Here's how the part is built. I have some questions about the finished solid (model axes, mm). Face numbers are marked on the shaded views. A direction names the side the tool comes from. Coordinates: 2 decimals unless noted, no trailing zeros. Order: outer loops, then holes, each group sorted by start corner. A loop starts at its lowest first (then second) coordinate and runs counter-clockwise, first axis right, second up. Notation, with made-up numbers: (58.5, 20.5) - (93.5, 20.5) arc R23 cw to (93.5, 28.5) - close; hole circle Ø4 at (-14.75, 59.25). An arc over 180 degrees is marked (long way). Answer in a Markdown table with one row per item. Add a question column.
Item 1: I want a section at C-C (x = 9). Please give me the cut outline in (y, z), plus the area to 3 significant figures.
Item 2: Will these pins go through, and if not, where does the flat tip stop? pin 1 Ø4 at (x, y) = (2.5, 3) entering from -Z; pin 2 Ø1.5 at (x, y) = (11, 12.5) entering from +Z; pin 3 Ø2 at (y, z) = (7, 5) entering from -X; pin 4 Ø5 at (x, z) = (13.5, 24) entering from -Y.
Item 3: I want a section at A-A (y = 0). Please give me the cut outline in (x, z) (3 decimals).
Item 4: Thinking about a two-plate mould opening in Z: for the marked faces 4, 5 and 6, which applies, +Z half, -Z half, draft (parallel to the pull), parting line (faces both ways), or undercut?
Item 5: If I drill on line 1 along Z through (x, y) = (-7, -14); line 2 along Y through (x, z) = (0, 24) (3 decimals); line 3 along Z through (x, y) = (7.5, -9), over which ranges is the centre line in solid material (lowest first)? Write a range as from..to.
Item 6: On a 3-axis mill with a long thin cutter (end or side, diameter ignored), from which of +Z, -Z, +X, -X, +Y, -Y can I reach the whole of each face in a straight line? I mean the marked faces 1, 2 and 3. Say none if no direction works.
Item 7: I want a section at D-D (z = 11.5). Please give me the cut outline in (x, y) (3 decimals), plus the area to 3 significant figures.
```python
from build123d import *

# Parameters (mm, degrees)
SZKIC1_R                    = 15.345
DODANIE_WYCI_GNI_CIE1_DEPTH = 30.5
SZKIC2_R                    = 11.5
DODANIE_WYCI_GNI_CIE2_DEPTH = 5.5
SZKIC3_R                    = 18
DODANIE_WYCI_GNI_CIE3_DEPTH = 0.5
SZKIC9_R                    = 18
DODANIE_WYCI_GNI_CIE6_DEPTH = 0.5
SZKIC6_R                    = 7
WYTNIJ_WYCI_GNI_CIE1_DEPTH  = 37


with BuildPart() as part:
    # Szkic1 → Dodanie-wyciągnięcie1 (new body)
    with BuildSketch(Plane.XY):
        Circle(SZKIC1_R)
    extrude(amount=DODANIE_WYCI_GNI_CIE1_DEPTH)

    # Szkic2 → Dodanie-wyciągnięcie2 (add)
    with BuildSketch(Plane.XY.offset(30.5)):
        Circle(SZKIC2_R)
    extrude(amount=DODANIE_WYCI_GNI_CIE2_DEPTH)

    # Szkic3 → Dodanie-wyciągnięcie3 (add)
    with BuildSketch(Plane.XY.offset(30.5)):
        Circle(SZKIC3_R)
    extrude(amount=-DODANIE_WYCI_GNI_CIE3_DEPTH)

    # Szkic9 → Dodanie-wyciągnięcie6 (add)
    with BuildSketch(Plane(origin=(0, 0, 0), x_dir=(-1, 0, 0), z_dir=(0, 0, -1))):
        Circle(SZKIC9_R)
    extrude(amount=-DODANIE_WYCI_GNI_CIE6_DEPTH)

    # Szkic6 → Wytnij-wyciągnięcie1 (cut, through all)
    with BuildSketch(Plane.XY.offset(36)):
        Circle(SZKIC6_R)
    extrude(amount=-WYTNIJ_WYCI_GNI_CIE1_DEPTH, mode=Mode.SUBTRACT)


solid = part.part
```
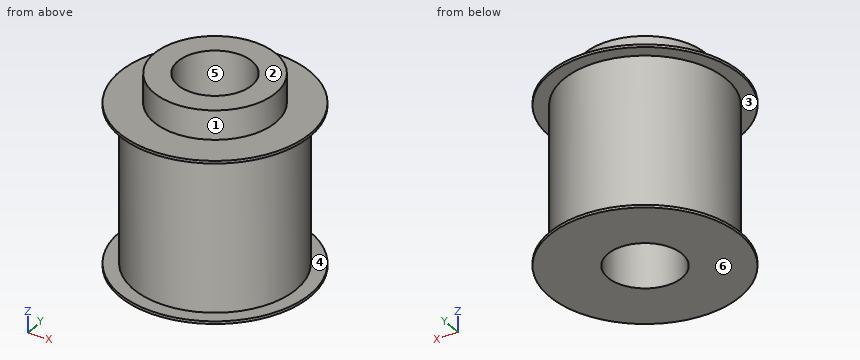
Values follow:
| question | item | result |
|---|---|---|
| 1 | outline | (-15.59, 0) - (15.59, 0) - (15.59, 0.5) - (12.43, 0.5) - (12.43, 30) - (15.59, 30) - (15.59, 30.5) - (7.16, 30.5) - (7.16, 36) - (-7.16, 36) - (-7.16, 30.5) - (-15.59, 30.5) - (-15.59, 30) - (-12.43, 30) - (-12.43, 0.5) - (-15.59, 0.5) - close |
| 1 | area | 843 mm^2 |
| 2 | pin 1 | passes through |
| 2 | pin 2 | stops at z = 30.5 |
| 2 | pin 3 | stops at x = -14.12 |
| 2 | pin 4 | stops at y = -10.7 |
| 3 | outline | (-18, 0) - (-7, 0) - (-7, 36) - (-11.5, 36) - (-11.5, 30.5) - (-18, 30.5) - (-18, 30) - (-15.345, 30) - (-15.345, 0.5) - (-18, 0.5) - close; (7, 0) - (18, 0) - (18, 0.5) - (15.345, 0.5) - (15.345, 30) - (18, 30) - (18, 30.5) - (11.5, 30.5) - (11.5, 36) - (7, 36) - close |
| 4 | face 4 | undercut |
| 4 | face 5 | draft |
| 4 | face 6 | -Z half |
| 5 | line 1 | z = 0..0.5, 30..30.5 |
| 5 | line 2 | y = -15.345..-7, 7..15.345 |
| 5 | line 3 | z = 0..30.5 |
| 6 | face 1 | +Z |
| 6 | face 2 | +Z, +X, -X, +Y, -Y |
| 6 | face 3 | none |
| 7 | outline | circle Ø30.69 at (0, 0); hole circle Ø14 at (0, 0) |
| 7 | area | 586 mm^2 |
